Read the model definition and answer for the solid it produces. Units are mm, in the model's axes. A direction names the side the tool comes from. Coordinates: 2 decimals unless noted, no trailing zeros. Write each loop counter-clockwise with the first axis right and the second up, starting at its lowest first coordinate (ties: lowest second). Pieces come first, ordered by that corner, then holes. Notation, with made-up numbers: (-34.75, -10) -> (-28.75, -10) arc R23 ccw to (-28.75, 13) -> close; hole circle Ø1 at (39, 48.5). An arc over 180 degrees is marked (long way). One line per item, written item: value. Start each with the question number.
1. Find section C-C, the plane x = 21.5. Write down the section's boundary in (y, z), and give its area (3 significant figures).
2. Given P1, Ø1.5, axis at x = 26.5, y = 12, coming from the -Z side; P2, Ø6, axis at y = 3, z = 33.5, coming from the +X side; P3, Ø6, axis at x = 24, y = 16.5, coming from the -Z side, each flat-ended and moving along its own axis, determine where each tip first touches the part or whether it passes through.
3. Find section D-D, the plane z = 33.75. Write down the section's boundary in (x, y), and give its area (3 significant figures).
4. Find section A-A, the plane z = 22.5. Write down the section's boundary in (x, y).
5. Consider line 1 along X through (y, z) = (17.75, 26); line 2 along X through (y, z) = (15.5, 42.5); line 3 along X through (y, z) = (5.5, 28.5). Determine where each line is inside the solid, lowest interval first.
6. For faces 1 (the flat face through (30.086, 10, 42)), 2 (the flat face through (40.086, 10, 42)), 3 (the flat face through (22.071, 9.86, 25.284)), determine the directions among +Z, -Z, +X, -X, +Y, -Y from which every point of the face is accessible in a straight line to the end or side of a thin tool.
7. Find section B-B, the plane y = 8. Write down the section's boundary in (x, z), and give its area (3 significant figures).
```python
from build123d import *

# Parameters (mm, degrees)
F1_DEPTH = 20


with BuildPart() as f1:
    # F0 (on Front) → F1 (new body)
    with BuildSketch(Plane.XZ):
        with BuildLine():
            ThreePointArc((17.5859551343, 19.07713693), (18.019843983, 22.9498427249), (19.2999951541, 26.6305115074))
            ThreePointArc((19.2999951541, 26.6305115074), (20.3740299114, 28.5539114993), (21.6811985158, 30.32713693))
            ThreePointArc((21.6811985158, 30.32713693), (25.4785218795, 33.7040718876), (30.0859551343, 35.8476467612))
            Line((30.0859551343, 35.8476467612), (30.0859551343, 41.0145478985))
            ThreePointArc((30.0859551343, 41.0145478985), (17.4968960349, 33.1083521304), (12.5859551343, 19.07713693))
            Line((12.5859551343, 19.07713693), (17.5859551343, 19.07713693))
        make_face()
        with BuildLine():
            Line((30.0859551343, 43.82713693), (30.0859551343, 41.0145478985))
            ThreePointArc((30.0859551343, 41.0145478985), (35.0859551343, 41.57713693), (40.0859551343, 41.0145478985))
            Line((40.0859551343, 41.0145478985), (40.0859551343, 43.82713693))
            Line((40.0859551343, 43.82713693), (30.0859551343, 43.82713693))
        make_face()
        with BuildLine():
            Line((30.0859551343, 41.0145478985), (30.0859551343, 35.8476467612))
            ThreePointArc((30.0859551343, 35.8476467612), (35.0859551343, 36.57713693), (40.0859551343, 35.8476467612))
            Line((40.0859551343, 35.8476467612), (40.0859551343, 41.0145478985))
            ThreePointArc((40.0859551343, 41.0145478985), (35.0859551343, 41.57713693), (30.0859551343, 41.0145478985))
        make_face()
        with BuildLine():
            ThreePointArc((48.4907117527, 30.32713693), (49.8138676132, 28.5290464732), (50.8973434351, 26.57713693))
            ThreePointArc((50.8973434351, 26.57713693), (52.1585837436, 22.921008984), (52.5859551343, 19.07713693))
            Line((52.5859551343, 19.07713693), (57.5859551343, 19.07713693))
            ThreePointArc((57.5859551343, 19.07713693), (52.6750142336, 33.1083521304), (40.0859551343, 41.0145478985))
            Line((40.0859551343, 41.0145478985), (40.0859551343, 35.8476467612))
            ThreePointArc((40.0859551343, 35.8476467612), (44.693388389, 33.7040718876), (48.4907117527, 30.32713693))
        make_face()
        with BuildLine():
            Line((19.2999951541, 26.6305115074), (24.9214912266, 23.8985655014))
            ThreePointArc((24.9214912266, 23.8985655014), (29.0725771912, 28.5851222957), (35.0859551343, 30.32713693))
            Line((35.0859551343, 30.32713693), (30.0859551343, 30.32713693))
            Line((30.0859551343, 30.32713693), (30.0859551343, 35.8476467612))
            ThreePointArc((30.0859551343, 35.8476467612), (25.4785218795, 33.7040718876), (21.6811985158, 30.32713693))
            ThreePointArc((21.6811985158, 30.32713693), (20.3740299114, 28.5539114993), (19.2999951541, 26.6305115074))
        make_face()
        with BuildLine():
            Line((30.0859551343, 30.32713693), (35.0859551343, 30.32713693))
            Line((35.0859551343, 30.32713693), (40.0859551343, 30.32713693))
            Line((40.0859551343, 30.32713693), (40.0859551343, 35.8476467612))
            ThreePointArc((40.0859551343, 35.8476467612), (35.0859551343, 36.57713693), (30.0859551343, 35.8476467612))
            Line((30.0859551343, 35.8476467612), (30.0859551343, 30.32713693))
        make_face()
        with BuildLine():
            Line((40.0859551343, 30.32713693), (35.0859551343, 30.32713693))
            ThreePointArc((35.0859551343, 30.32713693), (41.0993330773, 28.5851222957), (45.2504190419, 23.8985655014))
            Line((45.2504190419, 23.8985655014), (50.8973434351, 26.57713693))
            ThreePointArc((50.8973434351, 26.57713693), (49.8138676132, 28.5290464732), (48.4907117527, 30.32713693))
            ThreePointArc((48.4907117527, 30.32713693), (44.693388389, 33.7040718876), (40.0859551343, 35.8476467612))
            Line((40.0859551343, 35.8476467612), (40.0859551343, 30.32713693))
        make_face()
    extrude(amount=-F1_DEPTH)


solid = f1.part
```
Answer block:
1. outline: (0, 25.56) -> (20, 25.56) -> (20, 37.01) -> (0, 37.01) -> close
1. area: 229 mm2
2. P1: stops at z = 25.35
2. P2: stops at x = 54.47
2. P3: stops at z = 23.9
3. outline: (18.03, 0) -> (52.14, 0) -> (52.14, 20) -> (18.03, 20) -> close
3. area: 682 mm2
4. outline: (12.85, 0) -> (17.92, 0) -> (17.92, 20) -> (12.85, 20) -> close; (52.25, 0) -> (57.32, 0) -> (57.32, 20) -> (52.25, 20) -> close
5. line 1: x = 13.68 to 19.01, 20.6 to 26.22, 43.95 to 49.68, 51.16 to 56.49
5. line 2: x = 30.09 to 40.09
5. line 3: x = 14.65 to 28.94, 41.23 to 55.52
6. face 1: +Z, -X, +Y, -Y
6. face 2: +Z, +X, +Y, -Y
6. face 3: -Z, +Y, -Y
7. outline: (12.59, 19.08) -> (17.59, 19.08) arc R17.5 cw to (19.3, 26.63) -> (24.92, 23.9) arc R11.25 cw to (45.25, 23.9) -> (50.9, 26.58) arc R17.5 cw to (52.59, 19.08) -> (57.59, 19.08) arc R22.5 ccw to (40.09, 41.01) -> (40.09, 43.83) -> (30.09, 43.83) -> (30.09, 41.01) arc R22.5 ccw to start
7. area: 541 mm2
